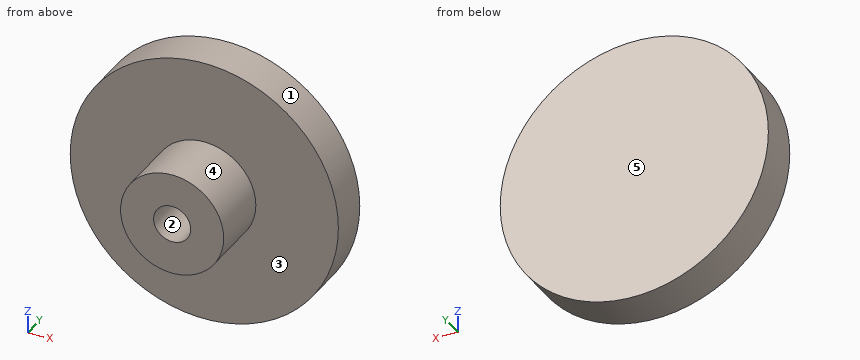
from build123d import *

# Parameters (mm, degrees)
F0_R     = 16.51
F1_DEPTH = 12.7
F2_R     = 2.286
F3_DEPTH = 7.62
F4_R     = 16.51
F4_R_2   = 6.35
F5_DEPTH = 7.62


with BuildPart() as f1:
    # F0 (on Front) → F1 (new body)
    with BuildSketch(Plane.XZ):
        Circle(F0_R)
    extrude(amount=-F1_DEPTH)

    # F2 (on face) → F3 (cut)
    with BuildSketch(Plane.XZ):
        Circle(F2_R)
    extrude(amount=-F3_DEPTH, mode=Mode.SUBTRACT)

    # F4 (on face) → F5 (cut)
    with BuildSketch(Plane.XZ):
        Circle(F4_R)
        Circle(F4_R_2, mode=Mode.SUBTRACT)
    extrude(amount=-F5_DEPTH, mode=Mode.SUBTRACT)


solid = f1.part
Read the model definition and answer for the solid it produces. Units are mm, in the model's axes. Face numbers are marked on the shaded views. A direction names the side the tool comes from. Give positions to 0.01 mm unless a question says otherwise; leave off trailing zeros. Write each loop counter-clockwise with the first axis right and the second up, starting at its lowest first coordinate (ties: lowest second). Pieces come first, ordered by that corner, then holes. Notation, with made-up numbers: (-21, -9.75) - (-1, -9.75) arc R25 cw to (-1, 8.25) - close; hole circle Ø4 at (42, -0.75). An arc over 180 degrees is marked (long way). Answer in a Markdown table with one row per item. Add a question column.
Item 1: Determine the mould class of the marked faces 1, 2 and 3 for opening direction X: pulls with the +X half, pulls with the -X half, needs draft (parallel to the pull), parting line crosses it, or undercut.
Item 2: Section A-A, the plane y = 3.5 is taken. Write down the section's boundary in (x, z).
Item 3: Section D-D, the plane y = 12.25 is taken. Write down the section's boundary in (x, z), and give its area (3 significant figures).
Item 4: Flat-ended cylindrical pins translate along their axes: P1, Ø6, axis at x = -6, y = 7.5, coming from the -Z side; P2, Ø2, axis at x = 6.5, y = 6.5, coming from the +Z side; P3, Ø1.5, axis at x = 9, y = 10, coming from the -Z side; P4, Ø3, axis at x = -4, z = 4.5, coming from the -Y side. Find the tip coordinate at first contact, or state that the pin passes through.
Item 5: Section C-C, the plane z = 0 is taken. Write down the section's boundary in (x, y), and give its area (3 significant figures).
Item 6: Section B-B, the plane x = 0 is taken. Write down the section's boundary in (y, z).
Item 7: Find the intervals of material crossed by L1, parallel to Z at x = 0, y = 3.75; L2, parallel to Y at x = 6.5, z = -2; L3, parallel to Z at x = 0, y = 11, in increasing order.
Item 8: A tool of negligible diameter and unlimited length cuts with its end or side. For the marked faces 4 and 5, from which of +Z, -Z, +X, -X, +Y, -Y can it reach the whole face along a straight path? Write none if from no direction.
Recorded:
| question | item | result |
|---|---|---|
| 1 | face 1 | parting line crosses it |
| 1 | face 2 | undercut |
| 1 | face 3 | needs draft |
| 2 | outline | circle Ø12.7 at (0, 0); hole circle Ø4.57 at (0, 0) |
| 3 | outline | circle Ø33.02 at (0, 0) |
| 3 | area | 856 mm2 |
| 4 | P1 | stops at z = -16.23 |
| 4 | P2 | stops at z = 3.17 |
| 4 | P3 | stops at z = -14.3 |
| 4 | P4 | stops at y = 0 |
| 5 | outline | (-16.51, 7.62) - (-6.35, 7.62) - (-6.35, 0) - (-2.29, 0) - (-2.29, 7.62) - (2.29, 7.62) - (2.29, 0) - (6.35, 0) - (6.35, 7.62) - (16.51, 7.62) - (16.51, 12.7) - (-16.51, 12.7) - close |
| 5 | area | 230 mm2 |
| 6 | outline | (0, -6.35) - (7.62, -6.35) - (7.62, -16.51) - (12.7, -16.51) - (12.7, 16.51) - (7.62, 16.51) - (7.62, 6.35) - (0, 6.35) - (0, 2.29) - (7.62, 2.29) - (7.62, -2.29) - (0, -2.29) - close |
| 7 | L1 | z = -6.35 to -2.29, 2.29 to 6.35 |
| 7 | L2 | y = 7.62 to 12.7 |
| 7 | L3 | z = -16.51 to 16.51 |
| 8 | face 4 | -Y |
| 8 | face 5 | +Z, -Z, +X, -X, +Y |
